Job drawing, mm, ordinate dimensions from the low corner. One solid piece. Round coordinates to 2 decimals unless told otherwise and drop trailing zeros. Write each loop counter-clockwise with the first axis right and the second up, starting at its lowest first coordinate (ties: lowest second). Pieces come first, ordered by that corner, then holes. Notation, with made-up numbers: (72, 20.5) - (94, 20.5) arc R4 cw to (94, 24.5) - close; hole circle Ø3 at (82.5, 18.5). An arc over 180 degrees is marked (long way). Write each question's results on one line, items separated by ' | '.
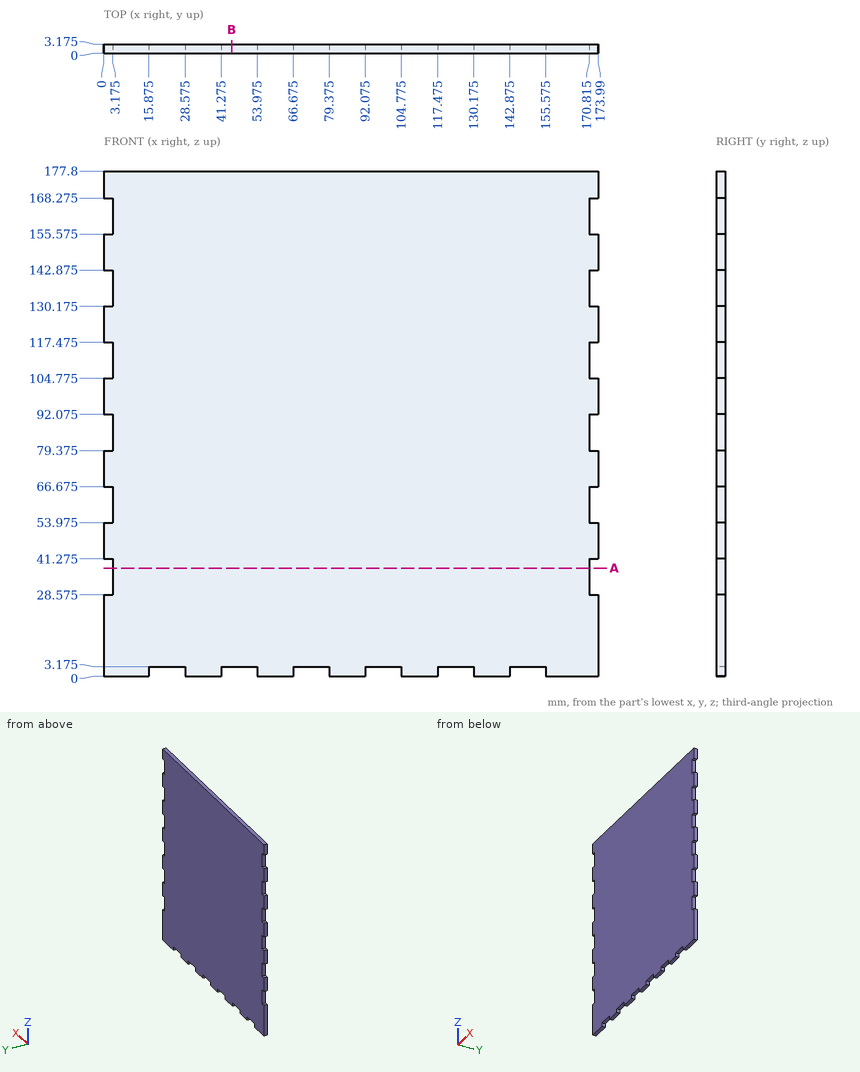
(1) Slice it at B-B, the plane x = 45. Write the cut outline in (y, z) (3 decimals).
Worked answers:
outline: (0, 3.175) - (3.175, 3.175) - (3.175, 177.8) - (0, 177.8) - close
(2) Drill centre lines: probe 1 along Z at (x, y) = (129, 2.6) (3 decimals); probe 2 along X at (y, z) = (2.8, 57.5) (3 decimals). Where is each one in solid material? Low to high. Write a range as [from, to].
Worked answers:
probe 1: z = [3.175, 177.8] | probe 2: x = [3.175, 170.815]
(3) Flat gauge pin, fed straight in: pin 1 Ø1 at (x, y) = (148.5, 1) entering from -Z (3 decimals). Where does the tip first touch, or does it go through?
Worked answers:
pin 1: stops at z = 3.175
(4) Slice it at A-A, the plane z = 38. Write the cut outline in (x, y) (3 decimals), and give its area (3 significant figures).
Worked answers:
outline: (3.175, 0) - (170.815, 0) - (170.815, 3.175) - (3.175, 3.175) - close | area: 532 mm2
